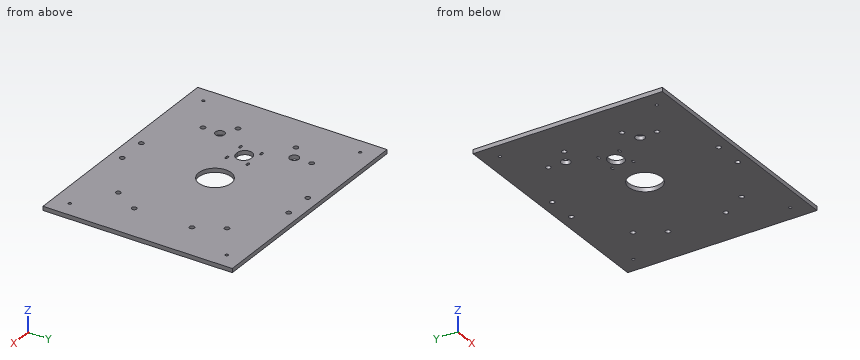
```python
from build123d import *

# Parameters (mm, degrees)
ESBO_O1_W                    = 350
ESBO_O1_H                    = 280
RESSALTO_EXTRUS_O1_DEPTH     = 6
ESBO_O2_R                    = 24
CORTE_EXTRUS_O1_DEPTH        = 225.189651858
FUROS_GUIA_COM_8_0MM1_D      = 8
FURO_DE_DI_METRO_3_2_3_2_1_D = 3.2
FURO_COM_FOLGA_DE_M121_D     = 13.5
ESBO_O9_R                    = 3.6
CORTE_EXTRUS_O2_DEPTH        = 10
FURO_DE_DI_METRO_4_2_4_2_1_D = 4.2
CORTE_EXTRUS_O3_DEPTH        = 225.189651858


with BuildPart() as part:
    # Esboço1 → Ressalto-extrusão1 (new body)
    with BuildSketch(Plane.XY.offset(5)):
        Rectangle(ESBO_O1_W, ESBO_O1_H)
    extrude(amount=-RESSALTO_EXTRUS_O1_DEPTH)

    # Esboço2 → Corte-extrusão1 (cut, through all)
    with BuildSketch(Plane.XY.offset(5)):
        Circle(ESBO_O2_R)
    extrude(amount=-CORTE_EXTRUS_O1_DEPTH, mode=Mode.SUBTRACT)

    # Furos-guia com Ø8.0mm1 (through all)
    with Locations(Plane.XY.offset(5)):
        with Locations((-67.5, 0)):
            Hole(FUROS_GUIA_COM_8_0MM1_D / 2)

    # Furo de diâmetro Ø3.2 (3.2)1 (through all)
    with Locations(Plane.XY.offset(5)):
        with Locations((-83, 15.5), (-83, -15.5), (-52, 15.5), (-52, -15.5)):
            Hole(FURO_DE_DI_METRO_3_2_3_2_1_D / 2)

    # Furo com folga de M121 (through all)
    with Locations(Plane.XY.offset(5)):
        with Locations((-95.262794416, 55), (-95.262794416, -55)):
            Hole(FURO_COM_FOLGA_DE_M121_D / 2)

    # Esboço9 → Corte-extrusão2 (cut)
    with BuildSketch(Plane.XY.offset(5)):
        with Locations((-95.75555539, 80.348451211)):
            Circle(ESBO_O9_R)
        with Locations(Location((-117.461577598, 42.752517916, 0), (0, 0, 180))):
            Circle(ESBO_O9_R)
        with Locations((21.706022208, 123.100969127)):
            Circle(ESBO_O9_R)
        with Locations(Location((-21.706022208, 123.100969127, 0), (0, 0, 180))):
            Circle(ESBO_O9_R)
        with Locations((117.461577598, 42.752517916)):
            Circle(ESBO_O9_R)
        with Locations(Location((95.75555539, 80.348451211, 0), (0, 0, 180))):
            Circle(ESBO_O9_R)
        with Locations((95.75555539, -80.348451211)):
            Circle(ESBO_O9_R)
        with Locations(Location((117.461577598, -42.752517916, 0), (0, 0, 180))):
            Circle(ESBO_O9_R)
        with Locations((-21.706022208, -123.100969127)):
            Circle(ESBO_O9_R)
        with Locations(Location((21.706022208, -123.100969127, 0), (0, 0, 180))):
            Circle(ESBO_O9_R)
        with Locations((-117.461577598, -42.752517916)):
            Circle(ESBO_O9_R)
        with Locations(Location((-95.75555539, -80.348451211, 0), (0, 0, 180))):
            Circle(ESBO_O9_R)
    extrude(amount=-CORTE_EXTRUS_O2_DEPTH, mode=Mode.SUBTRACT)

    # Furo de diâmetro Ø4.2 (4.2)1 (through all)
    with Locations(Plane.XY.offset(5)):
        with Locations((-151, 116), (151, 116), (151, -116), (-151, -116)):
            Hole(FURO_DE_DI_METRO_4_2_4_2_1_D / 2)

    # Esboço12 → Corte-extrusão3 (cut, through all)
    with BuildSketch(Plane.XY.offset(5)):
        with BuildLine():
            Line((-67.5, 11), (-64.5, 11))
            ThreePointArc((-64.5, 11), (-53.5, 0), (-64.5, -11))
            Line((-64.5, -11), (-67.5, -11))
            ThreePointArc((-67.5, -11), (-78.5, 0), (-67.5, 11))
        make_face()
        with BuildLine():
            Line((-83, 17.1), (-80, 17.1))
            ThreePointArc((-80, 17.1), (-78.4, 15.5), (-80, 13.9))
            Line((-80, 13.9), (-83, 13.9))
            ThreePointArc((-83, 13.9), (-84.6, 15.5), (-83, 17.1))
        make_face()
        with BuildLine():
            Line((-83, -13.9), (-80, -13.9))
            ThreePointArc((-80, -13.9), (-78.4, -15.5), (-80, -17.1))
            Line((-80, -17.1), (-83, -17.1))
            ThreePointArc((-83, -17.1), (-84.6, -15.5), (-83, -13.9))
        make_face()
        with BuildLine():
            Line((-52, 17.1), (-49, 17.1))
            ThreePointArc((-49, 17.1), (-47.4, 15.5), (-49, 13.9))
            Line((-49, 13.9), (-52, 13.9))
            ThreePointArc((-52, 13.9), (-53.6, 15.5), (-52, 17.1))
        make_face()
        with BuildLine():
            Line((-52, -13.9), (-49, -13.9))
            ThreePointArc((-49, -13.9), (-47.4, -15.5), (-49, -17.1))
            Line((-49, -17.1), (-52, -17.1))
            ThreePointArc((-52, -17.1), (-53.6, -15.5), (-52, -13.9))
        make_face()
    extrude(amount=-CORTE_EXTRUS_O3_DEPTH, mode=Mode.SUBTRACT)


solid = part.part
```
Verification items for the finished model (mm, model axes). Coordinates: 2 decimals unless noted, no trailing zeros. Loops run counter-clockwise (first coordinate to the right, second up) from the corner with the lowest first, then second, coordinate; pieces in that order, holes last. Notation, with made-up numbers: (43.25, -18.5) - (99.25, -18.5) arc R7 ccw to (99.25, -8.5) - close; hole circle Ø2 at (73, 86.25). An arc over 180 degrees is marked (long way). Put each result on its own line as item: value.
Item 1: Gauge pin test, flat end, axial feed: pin 1 Ø8.5 at (x, y) = (21.71, 123.1) entering from +Z. Record the tip position at first contact, or that the pin passes through.
Conclusion:
pin 1: stops at z = 5
Item 2: Scan lines: line 1 along Y through (x, z) = (151, 2.3); line 2 along Y through (x, z) = (-151.5, 1.6); line 3 along X through (y, z) = (-5.5, 2). Record each from-to range of solid material in increasing order.
Conclusion:
line 1: y = -140 to -118.1, -113.9 to 113.9, 118.1 to 140
line 2: y = -140 to -118.04, -113.96 to 113.96, 118.04 to 140
line 3: x = -175 to -77.03, -54.97 to -23.36, 23.36 to 175
Item 3: Section check D-D (z = -0.1). Give the number of separate pieces and of enclosed holes in the cut face, then the cut area to 3 significant figures.
Conclusion:
separate pieces: 1
enclosed holes: 24
area: 94,800 mm2
Item 4: Section check B-B (y = 0). Enter the section's corners in (x, z).
Conclusion:
outline: (-175, -1) - (-78.5, -1) - (-78.5, 5) - (-175, 5) - close; (-53.5, -1) - (-24, -1) - (-24, 5) - (-53.5, 5) - close; (24, -1) - (175, -1) - (175, 5) - (24, 5) - close
Item 5: Section check C-C (y = -55). Enter the section's corners in (x, z).
Conclusion:
outline: (-175, -1) - (-102.01, -1) - (-102.01, 5) - (-175, 5) - close; (-88.51, -1) - (175, -1) - (175, 5) - (-88.51, 5) - close
Item 6: Section check A-A (x = 0). Enter the section's corners in (y, z), then the cut area to 3 significant figures.
Conclusion:
outline: (-140, -1) - (-24, -1) - (-24, 5) - (-140, 5) - close; (24, -1) - (140, -1) - (140, 5) - (24, 5) - close
area: 1,390 mm2
